from build123d import *

# Parameters (mm, degrees)
F0_W     = 101.6
F0_H     = 101.6
F1_DEPTH = 13.208
F2_R     = 14.002831
F3_DEPTH = 8.636
F5_W     = 65.857943
F5_H     = 65.231863
F6_DEPTH = 5.588
F7_R     = 5.08


with BuildPart() as f1:
    # F0 (on Top) → F1 (new body)
    with BuildSketch(Plane.XY):
        Rectangle(F0_W, F0_H)
    extrude(amount=F1_DEPTH)

    # F2 (on face) → F3 (join)
    with BuildSketch(Plane(origin=(0, 0, 0), x_dir=(1, 0, 0), z_dir=(0, 0, -1))):
        Circle(F2_R)
    extrude(amount=F3_DEPTH)

    # F5 (on face) → F6 (join)
    with BuildSketch(Plane.XY.offset(13.208)):
        with Locations((-1.412789, -0.793302)):
            Rectangle(F5_W, F5_H)
    extrude(amount=F6_DEPTH)

    # F7
    f7_edges = [f1.edges().sort_by_distance(p)[0] for p in [
        (-50.8, 0, 0),
        (0, 50.8, 0),
        (50.8, 0, 0),
        (0, -50.8, 0),
    ]]
    fillet(f7_edges, radius=F7_R)


solid = f1.part
Source: CAD feature listing. Evaluate the final solid. Frame: model axes, mm. A direction names the side the tool comes from. Round coordinates to 2 decimals unless told otherwise and drop trailing zeros. Order: outer loops, then holes, each group sorted by start corner. A loop starts at its lowest first (then second) coordinate and runs counter-clockwise, first axis right, second up. Notation, with made-up numbers: (46.5, 81) - (76.5, 81) arc R14 cw to (76.5, 92) - close; hole circle Ø8 at (64.25, 70). An arc over 180 degrees is marked (long way). Use a Markdown table: item, result. Add a question column.
1. Line query: probe 1 along Z at (x, y) = (14, 29.5); probe 2 along Z at (x, y) = (26, -39); probe 3 along Y at (x, z) = (-17.5, 14.75). Output: solid intervals per line, ascending.
2. Section query C-C (z = -4). Return the cut outline in (x, y).
3. Section query D-D (x = 0). Return the cut outline in (y, z), then the cut area to 3 significant figures.
4. Set-up query: faces 1 (the flat face through (-2, -33.409, 16)), 2 (the flat face through (-34.342, -1, 16)), 3 (the flat face through (31.516, -1, 16)), 4 (the flat face through (-11, 11, 0)). Return all of +Z, -Z, +X, -X, +Y, -Y with unobstructed straight access to the full face (end or side cutting, diameter ignored); none if empty.
5. Section query B-B (y = -11.5). Return the cut outline in (x, z).
6. Section query A-A (x = 28). Return the cut outline in (y, z), then the cut area to 3 significant figures.
7. First-contact query: pin 1 (8 mm diameter, centred on y = 25.5, z = 1.5, fed in from +X); pin 2 (3 mm diameter, centred on x = 20.5, y = -36, fed in from -Z); pin 3 (3 mm diameter, centred on y = 5.5, z = 17, fed in from -X); pin 4 (3 mm diameter, centred on x = 1, z = 15.5, fed in from -Y). Flat tips, straight axial feed; report the tip coordinate or a pass-through.
Derived:
| question | item | result |
|---|---|---|
| 1 | probe 1 | 0 to 18.8 |
| 1 | probe 2 | 0 to 13.21 |
| 1 | probe 3 | -33.41 to 31.82 |
| 2 | outline | circle Ø28.01 at (0, 0) |
| 3 | outline | (-50.8, 5.08) arc R5.08 ccw to (-45.72, 0) - (-14, 0) - (-14, -8.64) - (14, -8.64) - (14, 0) - (45.72, 0) arc R5.08 ccw to (50.8, 5.08) - (50.8, 13.21) - (31.82, 13.21) - (31.82, 18.8) - (-33.41, 18.8) - (-33.41, 13.21) - (-50.8, 13.21) - close |
| 3 | area | 1,940 mm2 |
| 4 | face 1 | +Z, +X, -X, -Y |
| 4 | face 2 | +Z, -X, +Y, -Y |
| 4 | face 3 | +Z, +X, +Y, -Y |
| 4 | face 4 | -Z |
| 5 | outline | (-50.8, 5.08) arc R5.08 ccw to (-45.72, 0) - (-7.99, 0) - (-7.99, -8.64) - (7.99, -8.64) - (7.99, 0) - (45.72, 0) arc R5.08 ccw to (50.8, 5.08) - (50.8, 13.21) - (31.52, 13.21) - (31.52, 18.8) - (-34.34, 18.8) - (-34.34, 13.21) - (-50.8, 13.21) - close |
| 6 | outline | (-50.8, 5.08) arc R5.08 ccw to (-45.72, 0) - (45.72, 0) arc R5.08 ccw to (50.8, 5.08) - (50.8, 13.21) - (31.82, 13.21) - (31.82, 18.8) - (-33.41, 18.8) - (-33.41, 13.21) - (-50.8, 13.21) - close |
| 6 | area | 1,700 mm2 |
| 7 | pin 1 | x = 50.8 |
| 7 | pin 2 | z = 0 |
| 7 | pin 3 | x = -34.34 |
| 7 | pin 4 | y = -33.41 |
